Read the model definition and answer for the solid it produces. Units are mm, in the model's axes. Give positions to 0.01 mm unless a question says otherwise; leave off trailing zeros. Write each loop counter-clockwise with the first axis right and the second up, starting at its lowest first coordinate (ties: lowest second). Pieces come first, ordered by that corner, then holes. Notation, with made-up numbers: M 17.25,6.25 L 34.25,6.25 A16 ccw 34.25,32.25 Z; hole C 1,4.5 d3. An arc over 180 degrees is marked long. Write each question's results on one line, items separated by ' | '. Start each with the question number.
```python
from build123d import *

# Parameters (mm, degrees)
SKETCH_3_R          = 0.15
SKETCH_4_R          = 0.223077301
SKETCH_4_R_2        = 0.1
CUT_EXTRUDE_1_DEPTH = 3


with BuildPart() as part:
    # Эскиз1 → Повернуть1 (revolve)
    with BuildSketch(Plane.XY):
        with BuildLine():
            Line((0, 0), (0, 0.3))
            add(Edge.make_bspline(
                [(0, 0.3), (0.11509679, 0.551800246), (0.767947767, 0.661200883), (1.447067915, 0.470950787), (1.985552848, 0.226242678), (2, 0)],
                knots=[0, 0, 0, 0, 0.344144109, 0.722890882, 1, 1, 1, 1], degree=3))
            Line((2, 0), (0, 0))
        make_face()
    revolve(axis=Axis((0, 0, 0), (1, 0, 0)))

    # По траектории1: sweep along a path in Эскиз2
    with BuildLine(Plane.XY) as sweep_1_path:
        Line((0, 0.12), (-81.381966011, 0.12))
        ThreePointArc((-81.381966011, 0.12), (-81.907697123, 0.269349192), (-82.276393202, 0.672786405))
        Line((-82.276393202, 0.672786405), (-82.723606798, 1.567213595))
        ThreePointArc((-82.723606798, 1.567213595), (-83.092302877, 1.970650808), (-83.618033989, 2.12))
        Line((-83.618033989, 2.12), (-88, 2.12))
    # Эскиз3 → По траектории1 (sweep)
    with BuildSketch(Plane.ZY):
        with Locations((0, 0.12)):
            Circle(SKETCH_3_R)
    sweep_1 = sweep(path=sweep_1_path.line)

    # Эскиз4 → Вырез-Вытянуть1 (cut)
    with BuildSketch(Plane.ZY.offset(88)):
        with Locations((0, 2.12)):
            Circle(SKETCH_4_R)
        with Locations((0, 2.12)):
            Circle(SKETCH_4_R_2, mode=Mode.SUBTRACT)
    cut_extrude_1 = extrude(amount=-CUT_EXTRUDE_1_DEPTH, mode=Mode.SUBTRACT)

    # Зеркальное отражение3: По траектории1, Вырез-Вытянуть1 across plane
    add(sweep_1.mirror(Plane.ZX))
    add(cut_extrude_1.mirror(Plane.ZX), mode=Mode.SUBTRACT)


solid = part.part
```
Item 1: Straight lines are drawn through the part: line 1 (Y direction, x = -42.5, z = -0.05); line 2 (Z direction, x = -14, y = 0.05); line 3 (X direction, y = 1.15, z = 0.1). For each, find the intervals that lie inside material, in ascending order.
Item 2: Section A-A, the plane x = -58.5 is taken. Determine the outline of the cut face in (y, z).
Item 3: Given P1, Ø0.5, axis at y = 0, z = 0, coming from the -X side; P2, Ø1.5, axis at x = -44, y = -2, coming from the -Z side, each flat-ended and moving along its own axis, determine where each tip first touches the part or whether it passes through.
Worked out:
1) line 1: y = -0.26 to 0.26 | line 2: z = -0.13 to 0.13 | line 3: x = -82.64 to -82.39
2) outline: M 0,-0.09 A0.15 ccw long 0,0.09 A0.15 ccw long Z
3) P1: stops at x = -82.13 | P2: passes through
